Can you work these out from the model? Positions are in its coordinate system, mm. Give positions to 0.01 mm unless a question says otherwise; leave off trailing zeros. Order: outer loops, then holes, each group sorted by start corner. A loop starts at its lowest first (then second) coordinate and runs counter-clockwise, first axis right, second up. Notation, with made-up numbers: M -7.75,2 L 10.25,2 A23 ccw 10.25,28 Z; hole C -22,-10.5 d7. An arc over 180 degrees is marked long. Use a Markdown table: item, result. Add a question column.
from build123d import *

# Parameters (mm, degrees)
F0_R     = 2.54
F1_DEPTH = 5.08


with BuildPart() as f1:
    # F0 (on Front) → F1 (new body)
    with BuildSketch(Plane.XZ):
        with BuildLine():
            ThreePointArc((-78.2961119143, 41.5283401708), (-71.4386747563, 40.3661663473), (-67.6296123648, 46.1856281841))
            ThreePointArc((-67.6296123648, 46.1856281841), (-68.160150528, 48.7265657925), (-69.6631128152, 50.8429161974))
            ThreePointArc((-69.6631128152, 50.8429161974), (-78.636900378, 50.5021277337), (-78.2961119143, 41.5283401708))
        make_face()
        with Locations((-73.9796123648, 46.1856281841)):
            Circle(F0_R, mode=Mode.SUBTRACT)
        with BuildLine():
            ThreePointArc((-69.6631128152, 50.8429161974), (-68.160150528, 48.7265657925), (-67.6296123648, 46.1856281841))
            ThreePointArc((-67.6296123648, 46.1856281841), (-71.4386747563, 40.3661663473), (-78.2961119143, 41.5283401708))
            Line((-78.2961119143, 41.5283401708), (-13.094079489, -18.9026537454))
            ThreePointArc((-13.094079489, -18.9026537454), (-13.4348682543, -9.9288660273), (-4.4610805236, -9.5880775949))
            Line((-4.4610805236, -9.5880775949), (-69.6631128152, 50.8429161974))
        make_face()
        with BuildLine():
            Line((107.3138316889, -113.1840666865), (-4.4610805236, -9.5880775949))
            ThreePointArc((-4.4610805236, -9.5880775949), (-2.9581183134, -11.7044279677), (-2.427580179, -14.24536551))
            ThreePointArc((-2.427580179, -14.24536551), (-6.2366424208, -20.0648272814), (-13.094079489, -18.9026537454))
            Line((-13.094079489, -18.9026537454), (98.6808325898, -122.4986427131))
            ThreePointArc((98.6808325898, -122.4986427131), (98.3400441261, -113.5248551502), (107.3138316889, -113.1840666865))
        make_face()
        with BuildLine():
            ThreePointArc((-2.427580179, -14.24536551), (-2.9581183134, -11.7044279677), (-4.4610805236, -9.5880775949))
            ThreePointArc((-4.4610805236, -9.5880775949), (-13.4348682543, -9.9288660273), (-13.094079489, -18.9026537454))
            ThreePointArc((-13.094079489, -18.9026537454), (-6.2366424208, -20.0648272814), (-2.427580179, -14.24536551))
        make_face()
        with Locations((-8.777580179, -14.24536551)):
            Circle(F0_R, mode=Mode.SUBTRACT)
        with BuildLine():
            ThreePointArc((109.3473321393, -117.8413546998), (108.8167939761, -115.3004170913), (107.3138316889, -113.1840666865))
            ThreePointArc((107.3138316889, -113.1840666865), (98.3400441261, -113.5248551502), (98.6808325898, -122.4986427131))
            ThreePointArc((98.6808325898, -122.4986427131), (105.5382697478, -123.6608165366), (109.3473321393, -117.8413546998))
        make_face()
        with Locations((102.9973321393, -117.8413546998)):
            Circle(F0_R, mode=Mode.SUBTRACT)
    extrude(amount=F1_DEPTH)


solid = f1.part
1. If we section it at B-B, the plane z = 24.5: List the corners of the cut face in (x, y) for me.
2. If we section it at C-C, the plane x = 31: List the corners of the cut face in (y, z) for me, then the cut area to 3 significant figures.
3. I need wall thicknesses on L1, parallel to Z at x = -46.5, y = -3.05; L2, parallel to X at y = -0.7, z = -103.5; L3, parallel to X at y = -4.6, z = -67. Which ranges of each line are inside material? Lowest first, please. Write a range as [from, to].
4. We'd pull the mould along Z, two halves only. Please class faces 1 (the face through (-78.541, -2.504, 50.603)), 2 (the face through (14, -5.08, -35)), 3 (the face through (-72.81, -2.5, 43.93)): +Z half, -Z half, draft (parallel to the pull), parting line (faces both ways), or undercut.
5. If we section it at A-A, the plane y = -2.15: List the corners of the cut face in (x, z) for me, then the cut area to 3 significant figures.
Geometry results:
| question | item | result |
|---|---|---|
| 1 | outline | M -59.92,-5.08 L -41.24,-5.08 L -41.24,0 L -59.92,0 Z |
| 2 | outline | M -5.08,-59.77 L 0,-59.77 L 0,-42.45 L -5.08,-42.45 Z |
| 2 | area | 88.0 mm^2 |
| 3 | L1 | z = [12.06, 29.37] |
| 3 | L2 | x = [78.18, 96.87] |
| 3 | L3 | x = [38.8, 57.48] |
| 4 | face 1 | parting line |
| 4 | face 2 | draft |
| 4 | face 3 | undercut |
| 5 | outline | M -78.3,41.53 L 98.68,-122.5 A6.35 ccw 107.31,-113.18 L -69.66,50.84 A6.35 ccw Z; hole C -73.98,46.19 d5.08; hole C -8.78,-14.25 d5.08; hole C 103,-117.84 d5.08 |
| 5 | area | 3,130 mm^2 |
